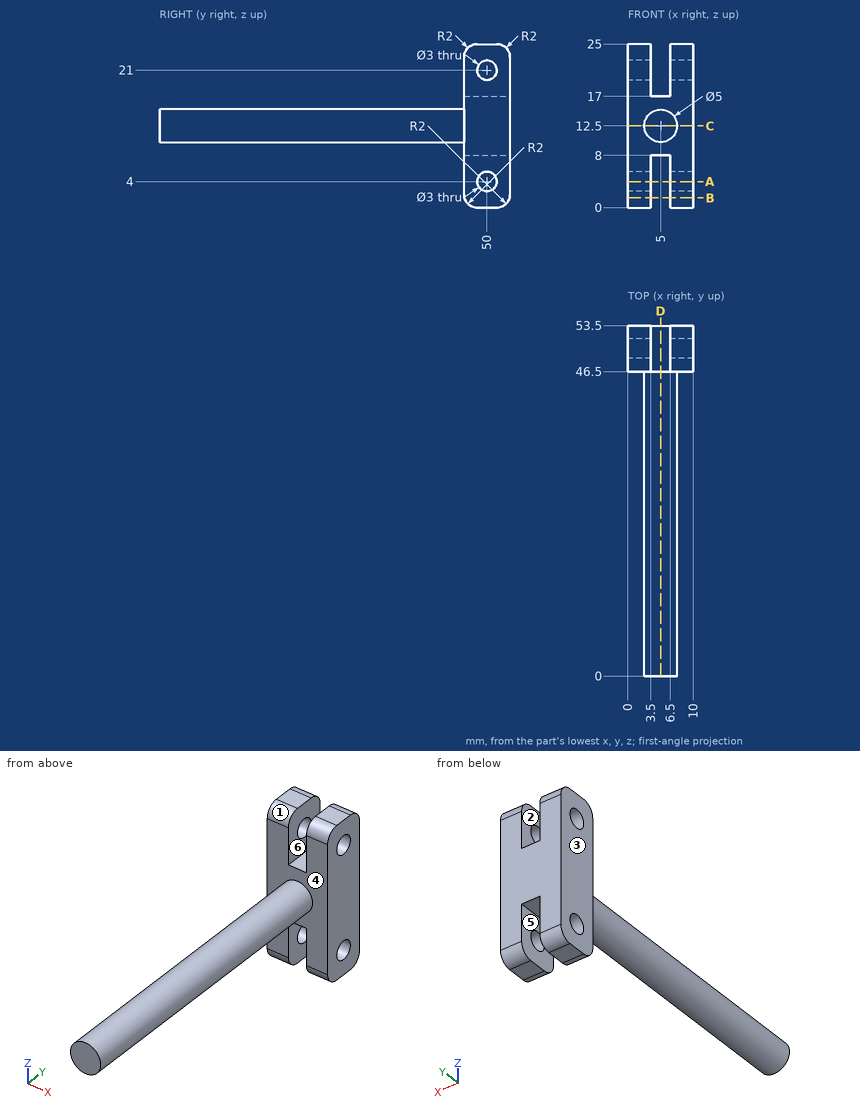
Answer from the drawing. Dimensions are ordinates in mm from the lowest x, y and z of the part. A direction names the side the tool comes from. Give positions to 0.01 mm unless a question says otherwise; leave off trailing zeros. Write each loop counter-clockwise with the first axis right and the second up, starting at its lowest first coordinate (ties: lowest second). Pieces come first, ordered by that corner, then holes. Notation, with made-up numbers: (35, 65.5) -> (93, 65.5) arc R21 ccw to (93, 84.5) -> close; hole circle Ø9 at (-36.75, -17). An arc over 180 degrees is marked (long way). One line per question, with ' | ' between items. Start each with the question number.
1. Section C-C (z = 12.5) is taken. Determine the outline of the cut face in (x, y).
2. Section A-A (z = 4) is taken. Determine the outline of the cut face in (x, y).
3. For the marked faces 4, 5 and 6, determine the directions among +Z, -Z, +X, -X, +Y, -Y from which every point of the face is accessible in a straight line to the end or side of a thin tool.
4. For a pull along X with two mould halves and no side action, classify the marked faces 1, 2 and 3 as pulls with the +X half, pulls with the -X half, needs draft (parallel to the pull), parting line crosses it, or undercut.
5. Find the intervals of material crossed by probe 1 along Z at (x, y) = (1, 50); probe 2 along Y at (x, z) = (2.65, 21); probe 3 along Y at (x, z) = (5.5, 9.5), in increasing order.
6. Section B-B (z = 1.5) is taken. Determine the outline of the cut face in (x, y), plus the area to 3 significant figures.
7. Section D-D (x = 5) is taken. Determine the outline of the cut face in (y, z).
8. Given pin 1 Ø0.9 at (x, y) = (4.5, 51.5) entering from +Z; pin 2 Ø5 at (x, z) = (2, 18.5) entering from -Y; pin 3 Ø1 at (x, y) = (7, 12.5) entering from +Z, each flat-ended and moving along its own axis, determine where each tip first touches the part or whether it passes through.
Response values:
1) outline: (0, 46.5) -> (2.5, 46.5) -> (2.5, 0) -> (7.5, 0) -> (7.5, 46.5) -> (10, 46.5) -> (10, 53.5) -> (0, 53.5) -> close
2) outline: (0, 46.5) -> (3.5, 46.5) -> (3.5, 48.5) -> (0, 48.5) -> close; (0, 51.5) -> (3.5, 51.5) -> (3.5, 53.5) -> (0, 53.5) -> close; (6.5, 46.5) -> (10, 46.5) -> (10, 48.5) -> (6.5, 48.5) -> close; (6.5, 51.5) -> (10, 51.5) -> (10, 53.5) -> (6.5, 53.5) -> close
3) face 4: -Y | face 5: -Z, +Y, -Y | face 6: +Z, +Y, -Y
4) face 1: needs draft | face 2: undercut | face 3: pulls with the -X half
5) probe 1: 0 to 2.5, 5.5 to 19.5, 22.5 to 25 | probe 2: 46.5 to 48.5, 51.5 to 53.5 | probe 3: 46.5 to 53.5
6) outline: (0, 46.56) -> (3.5, 46.56) -> (3.5, 53.44) -> (0, 53.44) -> close; (6.5, 46.56) -> (10, 46.56) -> (10, 53.44) -> (6.5, 53.44) -> close | area: 48.1 mm2
7) outline: (0, 10) -> (46.5, 10) -> (46.5, 8) -> (53.5, 8) -> (53.5, 17) -> (46.5, 17) -> (46.5, 15) -> (0, 15) -> close
8) pin 1: z = 17 | pin 2: y = 46.5 | pin 3: z = 14.5
